from build123d import *

# Parameters (mm, degrees)
BOSS_EXTRU_1_DEPTH = 2


with BuildPart() as part:
    # Esquisse1 → Boss.-Extru.1 (new body)
    with BuildSketch(Plane.XY):
        Polygon((-63.997372642, -108.680130338), (236.002627358, -108.680130338), (236.002627358, -98.108701767), (242.002627358, -98.108701767), (242.002627358, -87.537273195), (236.002627358, -87.537273195), (236.002627358, -76.965844624), (242.002627358, -76.965844624), (242.002627358, -66.394416052), (236.002627358, -66.394416052), (236.002627358, -55.822987481), (242.002627358, -55.822987481), (242.002627358, -45.25155891), (-69.997372642, -45.25155891), (-69.997372642, -55.822987481), (-63.997372642, -55.822987481), (-63.997372642, -66.394416052), (-69.997372642, -66.394416052), (-69.997372642, -76.965844624), (-63.997372642, -76.965844624), (-63.997372642, -87.537273195), (-69.997372642, -87.537273195), (-69.997372642, -98.108701767), (-63.997372642, -98.108701767), align=None)
    extrude(amount=-BOSS_EXTRU_1_DEPTH)


solid = part.part
Geometry: final body of the model. Coordinates: model frame, mm. Give positions to 0.01 mm unless a question says otherwise; leave off trailing zeros. Order: outer loops, then holes, each group sorted by start corner. A loop starts at its lowest first (then second) coordinate and runs counter-clockwise, first axis right, second up. Notation, with made-up numbers: (18, 11) -> (69, 11) arc R20 cw to (69, 21) -> close; hole circle Ø4 at (33, 18.25). An arc over 180 degrees is marked (long way). Answer as a JSON object with one key per item and string values.
Q1. First-contact query: pin 1 (0.6 mm diameter, centred on x = 239.5, z = -1.5, fed in from -Y); pin 2 (0.6 mm diameter, centred on y = -101.5, z = -1.5, fed in from -X); pin 3 (1 mm diameter, centred on y = -84.5, z = -0.5, fed in from +X). Flat tips, straight axial feed; report the tip coordinate or a pass-through.
Entries:
{"pin 1": "stops at y = -98.11", "pin 2": "stops at x = -64", "pin 3": "stops at x = 236"}
Q2. Section B-B (y = -102). Output: boundary loops of the cut face in (x, z).
Entries:
{"outline": "(-64, -2) -> (236, -2) -> (236, 0) -> (-64, 0) -> close"}
Q3. Material intervals for probe 1 along X at (y, z) = (-101, -1.65), sorted ascending.
Entries:
{"probe 1": "x = -64 to 236"}
Q4. Section A-A (z = -1.65). Output: boundary loops of the cut face in (x, y).
Entries:
{"outline": "(-70, -98.11) -> (-64, -98.11) -> (-64, -108.68) -> (236, -108.68) -> (236, -98.11) -> (242, -98.11) -> (242, -87.54) -> (236, -87.54) -> (236, -76.97) -> (242, -76.97) -> (242, -66.39) -> (236, -66.39) -> (236, -55.82) -> (242, -55.82) -> (242, -45.25) -> (-70, -45.25) -> (-70, -55.82) -> (-64, -55.82) -> (-64, -66.39) -> (-70, -66.39) -> (-70, -76.97) -> (-64, -76.97) -> (-64, -87.54) -> (-70, -87.54) -> close"}
